Autodesk Inventor part; units mm, degrees
ref_plane "YZ Plane" through (0, 0, 0) normal (1, 0, 0) x (0, 1, 0)
ref_plane "XZ Plane" through (0, 0, 0) normal (0, 1, 0) x (-1, 0, 0)
ref_plane "XY Plane" through (0, 0, 0) normal (0, 0, 1) x (1, 0, 0)
sketch "Эскиз1" plane through (0, 0, 0) normal (0, 0, 1) x (1, 0, 0)
  line L0 (0, 26) -> (22.5167, 13)
  line L1 (22.5167, 13) -> (22.5167, -13)
  line L2 (22.5167, -13) -> (0, -26)
  line L3 (0, -26) -> (-22.5167, -13)
  line L4 (-22.5167, -13) -> (-22.5167, 13)
  line L5 (-22.5167, 13) -> (0, 26)
  point P0 (0, 0)
  point P1 (0, 0)
  dimension "d0" = 52
extrude "Выдавливание1" add sketch "Эскиз1" along normal blind 18
sketch "Эскиз2" plane through (0, 0, 18) normal (0, 0, 1) x (1, 0, 0)
  circle A0 centre (0, 0) radius 16.6245
  dimension "d3" = 33.249
sketch "Эскиз3" plane through (0, 0, 0) normal (0, 0, -1) x (-1, 0, 0)
  circle A0 centre (0, 0) radius 21
  dimension "d4" = 42
extrude "Выдавливание2" add sketch "Эскиз3" along normal blind 40
extrude "Выдавливание3" add sketch "Эскиз2" along normal blind 32
sketch "Эскиз4" plane through (0, 0, 50) normal (0, 0, 1) x (1, 0, 0)
  circle A0 centre (0, 0) radius 8.25
  dimension "d9" = 16.5
sketch "Эскиз5" plane through (0, 0, -40) normal (0, 0, -1) x (-1, 0, 0)
  point P0 (0, 0)
  point P1 (0, 0)
hole "Отверстие1" at (0, 0, -40) direction (0, 0, 1) diameter 29.211 depth 32
extrude "Выдавливание4" cut sketch "Эскиз4" against normal through all
thread "Резьба1"
thread "Резьба2"
sketch "Эскиз6" plane through (0, 0, 0) normal (1, 0, 0) x (0, 1, 0)
  line L0 (26, 0) -> (26, 18)
  line L1 (13, 18) -> (26, 18)
  line L2 (26, 0) -> (13, 0)
  line L3 (26, 15.1132) -> (21, 18)
  line L4 (26, 2.8868) -> (21, 0)
  line L5 (0, -58) -> (0, 68)
  point P0 (0, 0)
  dimension "d25" = 21
  dimension "d26" = 30
  dimension "d27" = 30
revolve "Вращение1" cut sketch "Эскиз6" angle 360 about axis through (0, 0, -10) along (0, 0, 1)
sketch "Эскиз7" plane through (0, 0, 0) normal (0, 1, 0) x (-1, 0, 0)
  line L0 (-16.6245, 18) -> (-16.6245, 50)
  line L1 (21, 18) -> (-21, 18)
  line L2 (-15.6464, 24.7464) -> (-16.6245, 25.7245)
  line L3 (-15.5, 24.3929) -> (-15.5, 19.6)
  line L4 (-16.6245, 18) -> (16.6245, 18)
  arc A0 (-17.1, 18) -> (-15.5, 19.6) centre (-17.1, 19.6) ccw
  arc A1 (-15.5, 24.3929) -> (-15.6464, 24.7464) centre (-16, 24.3929) ccw
  line L5 (15.5, -9.6) -> (15.5, -12.5858)
  line L6 (15.2071, -13.2929) -> (14.6055, -13.8945)
  line L7 (14.6055, -8) -> (14.6055, -40)
  line L8 (-14.6055, -8) -> (14.6055, -8)
  line L9 (13.9, -8) -> (13.4971, -8)
  arc A2 (15.5, -9.6) -> (13.9, -8) centre (13.9, -9.6) ccw
  arc A3 (15.2071, -13.2929) -> (15.5, -12.5858) centre (14.5, -12.5858) ccw
  line L10 (-21, -10) -> (-20.5, -10)
  line L11 (-19.5, -11) -> (-19.5, -13)
  line L12 (-19.6464, -13.3536) -> (-21, -14.7071)
  arc A4 (-19.5, -11) -> (-20.5, -10) centre (-20.5, -11) ccw
  arc A5 (-19.6464, -13.3536) -> (-19.5, -13) centre (-20, -13) ccw
  line L13 (-21, 0) -> (-21, -40)
  line L14 (14.6055, -13.8945) -> (13.4971, -8)
  line L15 (-21, -10) -> (-21, -14.7071)
  line L16 (-16.6245, 25.7245) -> (-17.1, 18)
  line L17 (0, -58) -> (0, 68)
  point P0 (0, 0)
  point P1 (-15.5, 24.6)
  point P2 (-15.5, 18)
  point P3 (15.5, -8)
  point P4 (15.5, -13)
  dimension "d29" = 31
  dimension "d30" = 45
  dimension "d31" = 1.6
  dimension "d32" = 5
  dimension "d33" = 0.5
  dimension "d34" = 31
  dimension "d35" = 45
  dimension "d36" = 1.6
  dimension "d37" = 5
  dimension "d38" = 1
  dimension "d39" = 45
  dimension "d40" = 1
  dimension "d41" = 0.5
  dimension "d42" = 3
  dimension "d43" = 30
  dimension "d44" = 39
revolve "Вращение2" cut sketch "Эскиз7" angle 360 about axis through (0, 0, -10) along (0, 0, 1) contours A0 L16 L0 | L0 L2 A1 L3 A0 | L5 A3 L6 L7 A2 | L7 L14 L8 A2 | L10 A4 L11 A5 L12 L13
chamfer "Фаска1" distance 1.6 angle 45 1 edges at (-16.6245, 0, 50)
chamfer "Фаска2" distance 2 angle 45 2 edges at (-8.25, 0, 50) (21, 0, -40)
chamfer "Фаска3" distance 3 angle 45 1 edges at (0, -14.6055, -40)
properties material "Вода"
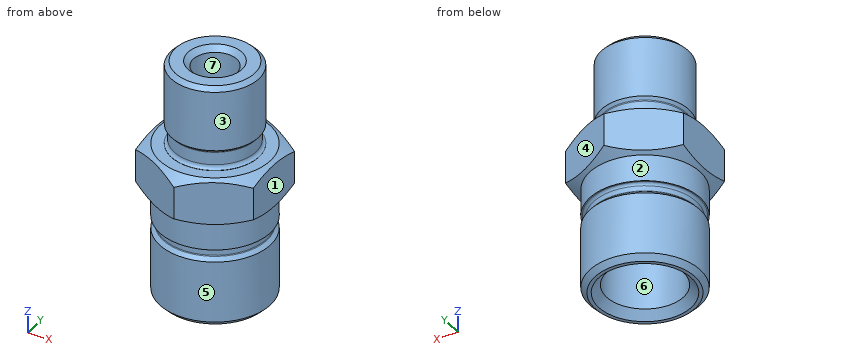
Model file for the job. Use its own axes, mm. Face numbers are marked on the shaded views. A direction names the side the tool comes from. Round coordinates to 2 decimals unless told otherwise and drop trailing zeros. Order: outer loops, then holes, each group sorted by start corner. A loop starts at its lowest first (then second) coordinate and runs counter-clockwise, first axis right, second up.
(1) Band-saw the part on A-A (z = -19.5). List the corners of the cut face in (x, y), then the cut area to 3 significant figures.
(2) Drill centre lines: line 1 (Y direction, x = 0, z = -11.55); line 2 (Y direction, x = 0, z = 29); line 3 (X direction, y = 0, z = -8.1). Where is each one in solid material? Low to high.
(3) Pull direction Y, two halves, no side cores. Call the marked faces 4, 5, 6 and 7: released by +Y, released by -Y, zero draft, split by the parting line, or undercut.
(4) Band-saw the part on B-B (z = 40). List the corners of the cut face in (x, y), then the cut area to 3 significant figures.
(5) Pin check, flat tips, straight feed: pin 1 (6 mm diameter, centred on y = -8, z = 26.5, fed in from -X); pin 2 (2 mm diameter, centred on x = 4, y = 5, fed in from -Z); pin 3 (19 mm diameter, centred on x = 0, y = 0, fed in from +Z); pin 4 (6 mm diameter, centred on x = -0.5, y = -13, fed in from -Z). Stop position of each tip, or through.
(6) 3-axis set-ups, long thin cutter, end or side, ignore diameter. For the marked faces 1, 2 and 3: which of +Z, -Z, +X, -X, +Y, -Y reach the whole face in a straight line?
Verdict:
1. outline: circle Ø42 at (0, 0); hole circle Ø29.21 at (0, 0)
1. area: 715 mm2
2. line 1: y = -19.5 to -15.5, 15.5 to 19.5
2. line 2: y = -16.62 to -8.25, 8.25 to 16.62
2. line 3: x = -21 to -14.61, 14.61 to 21
3. face 4: released by +Y
3. face 5: split by the parting line
3. face 6: undercut
3. face 7: undercut
4. outline: circle Ø33.25 at (0, 0); hole circle Ø16.5 at (0, 0)
4. area: 654 mm2
5. pin 1: stops at x = -15.85
5. pin 2: passes through
5. pin 3: stops at z = 49.25
5. pin 4: stops at z = -38.4
6. face 1: +Z, -Z, +X, +Y, -Y
6. face 2: -Z
6. face 3: +Z
